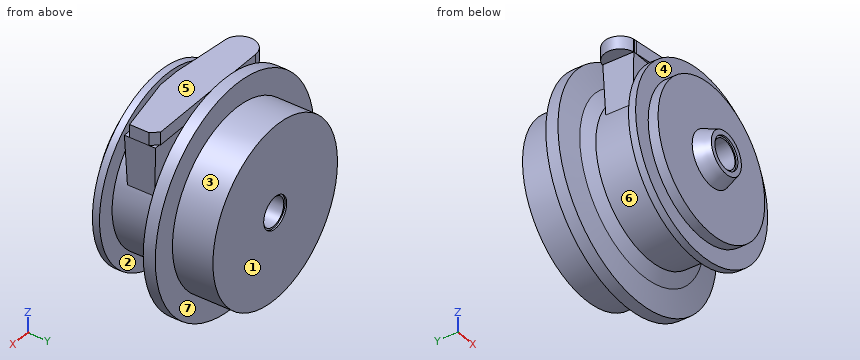
```python
from build123d import *

# Parameters (mm, degrees)
BOSS_EXTRUDE1_REACH      = 97.167
BOSS_EXTRUDE1_END_RADIUS = 28.847569448
SKETCH2_W                = 55
SKETCH2_H                = 12
BOSS_EXTRUDE1_DRAFT      = -2
BOSS_EXTRUDE2_DEPTH      = 5


with BuildPart() as part:
    # Sketch1 → Revolve1 (revolve)
    with BuildSketch(Plane.XY, mode=Mode.PRIVATE) as revolve1_sk:
        Polygon((5.51, 42.955132593), (5.51, -10.526859692), (6.21, -10.526859692), (6.21, -11.156859692), (8.117657505, -11.156859692), (10.386196058, -5.377232125), (28.847569448, -5.377232125), (28.847569448, -1.58033765), (35.664678952, -1.58033765), (35.664678952, 1.169396269), (28.847569448, 1.169396269), (28.847569448, 18.677058662), (33.66, 21.427260592), (42.91, 23.261015516), (42.91, 27.935132593), (33.66, 27.935132593), (33.66, 43.585132593), (6.21, 43.585132593), (6.21, 42.955132593), align=None)
    revolve(revolve1_sk.sketch.rotate(Axis((0, 28.345538502, 0), (0, -1, 0)), 180), axis=Axis((0, 28.345538502, 0), (0, -1, 0)))

    # Boss-Extrude1: up to this cylinder (the profile starts outside it)
    boss_extrude1_end = Plane(origin=(0, 10.956247, 0), z_dir=(0, 1, 0)) * Cylinder(BOSS_EXTRUDE1_END_RADIUS, 253.029138896, mode=Mode.PRIVATE)



with BuildPart() as boss_extrude1_long_prism_1:
    # Sketch2 → Boss-Extrude1 (the long prism of profile 1, to be tilted and cut off)
    with BuildSketch(Plane.XY.offset(30)):
        with Locations((0, 10.956246724)):
            Rectangle(SKETCH2_W, SKETCH2_H)
    extrude(amount=-BOSS_EXTRUDE1_REACH)
    boss_extrude1_tool1_sides = [boss_extrude1_long_prism_1.faces().sort_by_distance(p)[0] for p in [
        (0, 16.956246724, -18.5835),
        (-27.5, 10.956246724, -18.5835),
        (0, 4.956246724, -18.5835),
        (27.5, 10.956246724, -18.5835),
    ]]
    draft(boss_extrude1_tool1_sides, Plane.XY.offset(30), BOSS_EXTRUDE1_DRAFT)  # the draft: side faces tilted about the start plane


with BuildPart() as part_1:
    add(part.part)
    boss_extrude1_tool1 = boss_extrude1_long_prism_1.part - boss_extrude1_end
    add(boss_extrude1_tool1.solids().sort_by_distance((0, 10.956247, 30))[0])

    # Sketch3 → Boss-Extrude2 (add)
    with BuildSketch(Plane.XY.offset(30)):
        with BuildLine():
            ThreePointArc((-27.18192553, 4.956246724), (-26.694955, 4.898123787), (-26.204912516, 4.878708906))
            Line((-26.204912516, 4.878708906), (-4.504702211, 2.425132726))
            Line((-4.504702211, 2.425132726), (4.504702211, 2.425132726))
            Line((4.504702211, 2.425132726), (27.5, 6.956827348))
            Line((27.5, 6.956827348), (27.5, 14.431115524))
            Line((27.5, 14.431115524), (25.099356835, 17.26707076))
            Line((25.099356835, 17.26707076), (-26.204912516, 17.26707076))
            ThreePointArc((-26.204912516, 17.26707076), (-32.364772816, 11.724041467), (-27.5, 5.01561109))
            Line((-27.5, 5.01561109), (-27.5, 4.956246724))
            Line((-27.5, 4.956246724), (-27.18192553, 4.956246724))
        make_face()
    extrude(amount=BOSS_EXTRUDE2_DEPTH)


solid = part_1.part
```
Input: part model. Units: mm. Frame: model coordinates. Face numbers are marked on the shaded views. A direction names the side the tool comes from. Give positions to 0.01 mm unless a question says otherwise; leave off trailing zeros. Loops run counter-clockwise (first coordinate to the right, second up) from the corner with the lowest first, then second, coordinate; pieces in that order, holes last. Notation, with made-up numbers: M -12,-38.75 L 15,-38.75 A21 ccw 15,-21.75 Z; hole C -6.5,67.25 d7. An arc over 180 degrees is marked long. Answer as CSV lines item,"result". Start each with the question number.
1. Reachability of the marked faces 4, 5, 6 and 7 from +Z, -Z, +X, -X, +Y, -Y: full face, straight path, thin tool, end or side. Return the list, or none.
2. Section B-B on x = -31. State how many separate pieces and enclosed holes the cut face has, plus the area to 3 significant figures.
3. Section A-A on y = 26.5. Return loops of the section in (x, z).
4. Line query: L1, parallel to Z at x = 0, y = 3; L2, parallel to Z at x = 0, y = 43.2; L3, parallel to Z at x = 0, y = 12.5. Output: solid intervals per line, ascending.
5. Pull-direction query (Y, two-part tool) for the marked faces 1, 2 and 3; classes: released by +Y, released by -Y, zero draft, split by the parting line, or undercut.
6. Pin query (flat end, axial travel): P1, Ø5.5, axis at x = 0, z = 33, coming from the -Y side; P2, Ø6, axis at x = -3, y = 9, coming from the -Z side; P3, Ø1, axis at y = 15.5, z = 7.5, coming from the -X side; P4, Ø6, axis at x = -1.5, z = -1.5, coming from the +Y side. Return the tip coordinate at first contact, or that it passes through.
Computed values:
1,face 4,"-Y"
1,face 5,"+Z, +X, -X"
1,face 6,"none"
1,face 7,"+Y"
2,separate pieces,"3"
2,enclosed holes,"0"
2,area,"932 mm²"
3,outline,"C 0,0 d85.82; hole C 0,0 d11.02"
4,L1,"z = -28.85 to -5.51, 5.51 to 28.85, 30 to 35"
4,L2,"z = -33.66 to -6.21, 6.21 to 33.66"
4,L3,"z = -28.85 to -5.51, 5.51 to 35"
5,face 1,"released by +Y"
5,face 2,"undercut"
5,face 3,"zero draft"
6,P1,"stops at y = -1.58"
6,P2,"stops at z = -28.85"
6,P3,"stops at x = -27.99"
6,P4,"passes through"
